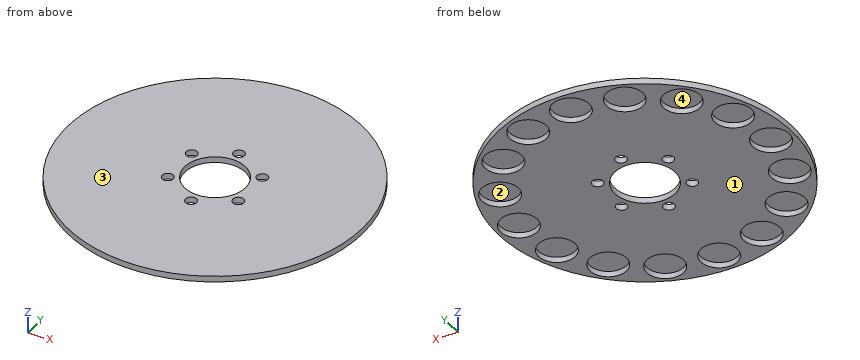
from build123d import *

# Parameters (mm, degrees)
ESQUISSE1_R        = 80
ESQUISSE1_R_2      = 3
ESQUISSE1_R_3      = 16.5
ESQUISSE1_R_4      = 10
BOSS_EXTRU_1_DEPTH = 3.2
BOSS_EXTRU_2_START = -0.2
ESQUISSE2_R        = 80
ESQUISSE2_R_2      = 53.253598624
BOSS_EXTRU_2_DEPTH = 0.2


with BuildPart() as part:
    # Esquisse1 → Boss.-Extru.1 (new body)
    with BuildSketch(Plane.XY):
        Circle(ESQUISSE1_R)
        with Locations((0, 22)):
            Circle(ESQUISSE1_R_2, mode=Mode.SUBTRACT)
        Circle(ESQUISSE1_R_3, mode=Mode.SUBTRACT)
        with Locations((19.052558883, 11)):
            Circle(ESQUISSE1_R_2, mode=Mode.SUBTRACT)
        with Locations((19.052558883, -11)):
            Circle(ESQUISSE1_R_2, mode=Mode.SUBTRACT)
        with Locations((0, -22)):
            Circle(ESQUISSE1_R_2, mode=Mode.SUBTRACT)
        with Locations((-19.052558883, -11)):
            Circle(ESQUISSE1_R_2, mode=Mode.SUBTRACT)
        with Locations((-19.052558883, 11)):
            Circle(ESQUISSE1_R_2, mode=Mode.SUBTRACT)
        with Locations((0, 68)):
            Circle(ESQUISSE1_R_4, mode=Mode.SUBTRACT)
        with Locations((26.022473401, 62.823808211)):
            Circle(ESQUISSE1_R_4, mode=Mode.SUBTRACT)
        with Locations((48.083261121, 48.083261121)):
            Circle(ESQUISSE1_R_4, mode=Mode.SUBTRACT)
        with Locations((62.823808211, 26.022473401)):
            Circle(ESQUISSE1_R_4, mode=Mode.SUBTRACT)
        with Locations((68, 0)):
            Circle(ESQUISSE1_R_4, mode=Mode.SUBTRACT)
        with Locations((62.823808211, -26.022473401)):
            Circle(ESQUISSE1_R_4, mode=Mode.SUBTRACT)
        with Locations((48.083261121, -48.083261121)):
            Circle(ESQUISSE1_R_4, mode=Mode.SUBTRACT)
        with Locations((26.022473401, -62.823808211)):
            Circle(ESQUISSE1_R_4, mode=Mode.SUBTRACT)
        with Locations((0, -68)):
            Circle(ESQUISSE1_R_4, mode=Mode.SUBTRACT)
        with Locations((-26.022473401, -62.823808211)):
            Circle(ESQUISSE1_R_4, mode=Mode.SUBTRACT)
        with Locations((-48.083261121, -48.083261121)):
            Circle(ESQUISSE1_R_4, mode=Mode.SUBTRACT)
        with Locations((-62.823808211, -26.022473401)):
            Circle(ESQUISSE1_R_4, mode=Mode.SUBTRACT)
        with Locations((-68, 0)):
            Circle(ESQUISSE1_R_4, mode=Mode.SUBTRACT)
        with Locations((-62.823808211, 26.022473401)):
            Circle(ESQUISSE1_R_4, mode=Mode.SUBTRACT)
        with Locations((-48.083261121, 48.083261121)):
            Circle(ESQUISSE1_R_4, mode=Mode.SUBTRACT)
        with Locations((-26.022473401, 62.823808211)):
            Circle(ESQUISSE1_R_4, mode=Mode.SUBTRACT)
    extrude(amount=BOSS_EXTRU_1_DEPTH)

    # Esquisse2 → Boss.-Extru.2 (add)
    with BuildSketch(Plane.XY.offset(3.2).offset(BOSS_EXTRU_2_START)):
        Circle(ESQUISSE2_R)
        Circle(ESQUISSE2_R_2, mode=Mode.SUBTRACT)
    extrude(amount=BOSS_EXTRU_2_DEPTH)


solid = part.part
Build history of the part. All positions in model axes, mm. Face numbers are marked on the shaded views. A direction names the side the tool comes from. Round coordinates to 2 decimals unless told otherwise and drop trailing zeros. Write each loop counter-clockwise with the first axis right and the second up, starting at its lowest first coordinate (ties: lowest second). Pieces come first, ordered by that corner, then holes. Notation, with made-up numbers: (6, 69) -> (55, 69) arc R15 ccw to (55, 79) -> close; hole circle Ø6 at (29.25, 59.5). An arc over 180 degrees is marked (long way). Use one line per item in the form item = value.
Q1. Drop flat-ended pins along their axis: P1, Ø16, axis at x = 0, y = -67, coming from the -Z side; P2, Ø1.5, axis at x = 46.5, z = 0.5, coming from the -Y side; P3, Ø1.5, axis at x = 43, z = 0.5, coming from the +Y side. Give the stop position or say it passes through.
Conclusion:
P1 = 3
P2 = -65.63
P3 = 67.93
Q2. Drill centre lines: L1, parallel to X at y = -68, z = 1.25; L2, parallel to Y at x = 9, z = 2.85; L3, parallel to X at y = 54.5, z = 2.05. Where is each one in solid material? Low to high.
Conclusion:
L1 = -42.14 to -34.58, -17.47 to -10, 10 to 17.47, 34.58 to 42.14
L2 = -79.49 to -72.36, -63.64 to -13.83, 13.83 to 63.64, 72.36 to 79.49
L3 = -58.56 to -55.75, -40.41 to -31.56, -20.48 to 20.48, 31.56 to 40.41, 55.75 to 58.56
Q3. Band-saw the part on D-D, the plane x = 68. Write the cut outline in (y, z), then the cut area to 3 significant figures.
Conclusion:
outline = (-42.14, 0) -> (-34.58, 0) -> (-34.58, 3) -> (-17.47, 3) -> (-17.47, 0) -> (-10, 0) -> (-10, 3) -> (10, 3) -> (10, 0) -> (17.47, 0) -> (17.47, 3) -> (34.58, 3) -> (34.58, 0) -> (42.14, 0) -> (42.14, 3.2) -> (-42.14, 3.2) -> close
area = 107 mm²
Q4. Band-saw the part on C-C, the plane y = -31.5. Write the cut outline in (x, z).
Conclusion:
outline = (-73.54, 0) -> (-71.19, 0) -> (-71.19, 3) -> (-54.46, 3) -> (-54.46, 0) -> (54.46, 0) -> (54.46, 3) -> (71.19, 3) -> (71.19, 0) -> (73.54, 0) -> (73.54, 3.2) -> (-73.54, 3.2) -> close
Q5. Two-plate mould, pull along Y, no slides. Class the marked faces 1 and 2: released by +Y, released by -Y, zero draft, split by the parting line, or undercut.
Conclusion:
face_1 = zero draft
face_2 = undercut
Q6. Tool access for the marked faces 3 and 4: list every direction of +Z, -Z, +X, -X, +Y, -Y with a clear straight run to the whole face (end or side of a thin tool).
Conclusion:
face_3 = +Z, +X, -X, +Y, -Y
face_4 = -Z
Q7. Band-saw the part on B-B, the plane z = 2.3. State how many separate pieces and enclosed holes the cut face has, then the cut area to 3 significant figures.
Conclusion:
separate_pieces = 1
enclosed_holes = 23
area = 14,100 mm²
Q8. Band-saw the part on A-A, the plane x = 0. Write the cut outline in (y, z), then the cut area to 3 significant figures.
Conclusion:
outline = (-80, 0) -> (-78, 0) -> (-78, 3) -> (-58, 3) -> (-58, 0) -> (-25, 0) -> (-25, 3.2) -> (-80, 3.2) -> close; (-19, 0) -> (-16.5, 0) -> (-16.5, 3.2) -> (-19, 3.2) -> close; (16.5, 0) -> (19, 0) -> (19, 3.2) -> (16.5, 3.2) -> close; (25, 0) -> (58, 0) -> (58, 3) -> (78, 3) -> (78, 0) -> (80, 0) -> (80, 3.2) -> (25, 3.2) -> close
area = 248 mm²
